```python
from build123d import *

# Parameters (mm, degrees)
SKETCH1_W                    = 25
SKETCH1_H                    = 46
BASE_FLANGE1_DEPTH           = 4.55422
EDGE_FLANGE2_STRIP_W         = 27.74188
EDGE_FLANGE2_STRIP_H         = 4.55422
EDGE_FLANGE2_STRIP_CUT_DEPTH = 46
EDGE_FLANGE2_DEPTH           = 46
EDGE_FLANGE3_STRIP_W         = 27.74188
EDGE_FLANGE3_STRIP_H         = 4.55422
EDGE_FLANGE3_STRIP_CUT_DEPTH = 46
EDGE_FLANGE3_DEPTH           = 46
FILLET1_R                    = 6
M6_CLEARANCE_HOLE1_D         = 6.6
CUT_EXTRUDE1_DEPTH           = 76.830940915


# Sheet-metal steps are written as plain solids
with BuildPart() as part:
    # Sketch1 → Base-Flange1 (new body)
    with BuildSketch(Plane.XY):
        with Locations((-12.5, 0)):
            Rectangle(SKETCH1_W, SKETCH1_H)
    extrude(amount=-BASE_FLANGE1_DEPTH)

    # Edge-Flange2 strip (across the edge) → Edge-Flange2 strip cut (cut)
    with BuildSketch(Plane(origin=(0, -23, 0), x_dir=(-1, 0, 0), z_dir=(0, 1, 0))):
        with Locations((-4.55422, -2.27711)):
            Rectangle(EDGE_FLANGE2_STRIP_W, EDGE_FLANGE2_STRIP_H)
    extrude(amount=EDGE_FLANGE2_STRIP_CUT_DEPTH, mode=Mode.SUBTRACT)

    # Edge-Flange2 section (across the edge) → Edge-Flange2 (add)
    with BuildSketch(Plane(origin=(0, -23, 0), x_dir=(-1, 0, 0), z_dir=(0, 1, 0))):
        with BuildLine():
            Line((0, 4.7625), (0, 33.44578))
            Line((0, 33.44578), (4.55422, 33.44578))
            Line((4.55422, 33.44578), (4.55422, 4.7625))
            ThreePointArc((4.55422, 4.7625), (5.949123955, 1.394903955), (9.31672, 0))
            Line((9.31672, 0), (9.31672, -4.55422))
            ThreePointArc((9.31672, -4.55422), (2.72880411, -1.82541589), (0, 4.7625))
        make_face()
    extrude(amount=EDGE_FLANGE2_DEPTH)

    # Edge-Flange3 strip (across the edge) → Edge-Flange3 strip cut (cut)
    with BuildSketch(Plane(origin=(0, 23, 33.44578), x_dir=(0, 0, -1), z_dir=(0, -1, 0))):
        with Locations((-4.55422, -2.27711)):
            Rectangle(EDGE_FLANGE3_STRIP_W, EDGE_FLANGE3_STRIP_H)
    extrude(amount=EDGE_FLANGE3_STRIP_CUT_DEPTH, mode=Mode.SUBTRACT)

    # Edge-Flange3 section (across the edge) → Edge-Flange3 (add)
    with BuildSketch(Plane(origin=(0, 23, 33.44578), x_dir=(0, 0, -1), z_dir=(0, -1, 0))):
        with BuildLine():
            Line((0, 4.7625), (0, 29.44578))
            Line((0, 29.44578), (4.55422, 29.44578))
            Line((4.55422, 29.44578), (4.55422, 4.7625))
            ThreePointArc((4.55422, 4.7625), (5.949123955, 1.394903955), (9.31672, 0))
            Line((9.31672, 0), (9.31672, -4.55422))
            ThreePointArc((9.31672, -4.55422), (2.72880411, -1.82541589), (0, 4.7625))
        make_face()
    extrude(amount=EDGE_FLANGE3_DEPTH)

    # Fillet1
    fillet1_edges = [part.edges().sort_by_distance(p)[0] for p in [
        (29.44578, 23, 31.16867),
        (29.44578, -23, 31.16867),
        (-25, 23, -2.27711),
        (-25, -23, -2.27711),
    ]]
    fillet(fillet1_edges, radius=FILLET1_R)

    # M6 Clearance Hole1 (through all)
    with Locations(Plane.XY):
        with Locations((-16, 10), (-16, -10)):
            Hole(M6_CLEARANCE_HOLE1_D / 2)

    # Sketch12 → Cut-Extrude1 (cut, through all)
    with BuildSketch(Plane(origin=(-32.01422, 0, 33.44578), x_dir=(1, 0, 0), z_dir=(0, 0, 1))):
        with BuildLine():
            Line((43.66422, -8), (43.66422, 8))
            ThreePointArc((43.66422, 8), (50.01422, 14.35), (56.36422, 8))
            Line((56.36422, 8), (56.36422, -8))
            ThreePointArc((56.36422, -8), (50.01422, -14.35), (43.66422, -8))
        make_face()
    extrude(amount=-CUT_EXTRUDE1_DEPTH, mode=Mode.SUBTRACT)


solid = part.part
```
Work out the finished part from the listing and answer in its coordinate system (mm). A direction names the side the tool comes from. Round coordinates to 2 decimals unless told otherwise and drop trailing zeros. Loops run counter-clockwise (first coordinate to the right, second up) from the corner with the lowest first, then second, coordinate; pieces in that order, holes last.
(1) Each of these flat-tipped pins is pushed along its axis until it touches: P1, Ø4, axis at x = -16, y = -10, coming from the -Z side; P2, Ø7.5, axis at x = -16, y = 10, coming from the +Z side; P3, Ø9.5, axis at y = -5, z = 17, coming from the +X side; P4, Ø10, axis at y = 10, z = 14.5, coming from the -X side. Where does it stop, or does it pass through?
Computed values:
P1: passes through
P2: stops at z = 0
P3: stops at x = 0
P4: stops at x = -4.55
(2) The part is cut by section C-C, the plane x = 18. Give the vertices of the cut face in (y, z), and give its area (3 significant figures).
Computed values:
outline: (-23, 28.89) - (-14.35, 28.89) - (-14.35, 33.45) - (-23, 33.45) - close; (14.35, 28.89) - (23, 28.89) - (23, 33.45) - (14.35, 33.45) - close
area: 78.8 mm2
(3) The part is cut by section D-D, the plane y = -10. Give the vertices of the cut face in (x, z) (1 decimal), and give its area (3 significant figures).
Computed values:
outline: (-25, -4.6) - (-19.3, -4.6) - (-19.3, 0) - (-25, 0) - close; (-12.7, -4.6) - (-9.3, -4.6) arc R9.3 ccw to (0, 4.8) - (0, 24.1) arc R4.8 cw to (4.8, 28.9) - (12, 28.9) - (12, 33.4) - (4.8, 33.4) arc R9.3 ccw to (-4.6, 24.1) - (-4.6, 4.8) arc R4.8 cw to (-9.3, 0) - (-12.7, 0) - close; (24, 28.9) - (29.4, 28.9) - (29.4, 33.4) - (24, 33.4) - close
area: 288 mm2
(4) The mould has two halves that part along X. Classify faces 1 (the cylindrical face through (17.86, 14.35, 31.2)), 2 (the flat face through (-17, 0, 0)), 3 (the cylindrical face through (-1.9, 0.32, 30.64)), 4 (the flat face through (29.446, 0, 31)): pulls with the +X half, pulls with the -X half, needs draft (parallel to the pull), parting line crosses it, or undercut.
Computed values:
face 1: undercut
face 2: needs draft
face 3: pulls with the -X half
face 4: pulls with the +X half
(5) The part is cut by section A-A, the plane x = -16. Give the vertices of the cut face in (y, z).
Computed values:
outline: (-23, -4.55) - (-13.3, -4.55) - (-13.3, 0) - (-23, 0) - close; (-6.7, -4.55) - (6.7, -4.55) - (6.7, 0) - (-6.7, 0) - close; (13.3, -4.55) - (23, -4.55) - (23, 0) - (13.3, 0) - close
(6) Find the intervals of material crossed by L1, parallel to Y at x = -16, z = -3.2; L2, parallel to Y at x = 18, z = 29.5; L3, parallel to X at y = 13.5, z = 22, in increasing order.
Computed values:
L1: y = -23 to -13.3, -6.7 to 6.7, 13.3 to 23
L2: y = -23 to -14.35, 14.35 to 23
L3: x = -4.55 to 0
(7) For faces 5 (the flat face through (24.35, 0, 31)), 6 (the cylindrical face through (27.73, -21.2, 31.14)), 7 (the flat face through (0, 0, 14)), determine the directions among +Z, -Z, +X, -X, +Y, -Y from which every point of the face is accessible in a straight line to the end or side of a thin tool.
Computed values:
face 5: +Z, -Z
face 6: +Z, -Z, +X, -Y
face 7: -Z, +X, +Y, -Y
